Geometry: final body of the model. Coordinates: model frame, mm. Give positions to 0.01 mm unless a question says otherwise; leave off trailing zeros.
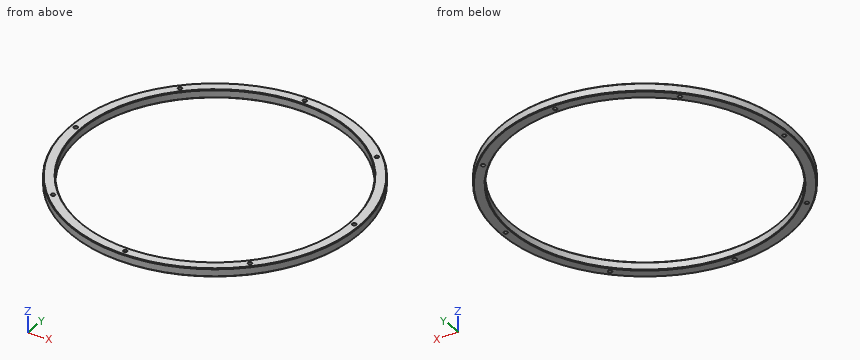
from build123d import *

# Parameters (mm, degrees)
SKETCH1_R             = 111.25
SKETCH1_R_2           = 103.25
EXTRUDE1_DEPTH        = 6.35
M3X0_5_TAPPED_HOLE1_D = 3
CIRPATTERN1_COUNT     = 8
CHAMFER1_SIZE         = 0.5


with BuildPart() as part:
    # Sketch1 → Extrude1 (new body)
    with BuildSketch(Plane.XY):
        Circle(SKETCH1_R)
        Circle(SKETCH1_R_2, mode=Mode.SUBTRACT)
    extrude(amount=EXTRUDE1_DEPTH)

    # M3x0.5 Tapped Hole1 (through all)
    with Locations(Plane.XY.offset(6.35)):
        with Locations((0, 107.125)):
            m3x0_5_tapped_hole1 = Hole(M3X0_5_TAPPED_HOLE1_D / 2)

    # CirPattern1: M3x0.5 Tapped Hole1 ×8 about axis
    cirpattern1_axis = Axis((0, 0, 0), (0, 0, 1))
    for i in range(1, CIRPATTERN1_COUNT):
        add(m3x0_5_tapped_hole1.rotate(cirpattern1_axis, i * 360 / CIRPATTERN1_COUNT), mode=Mode.SUBTRACT)

    # Chamfer1
    chamfer1_edges = [part.edges().sort_by_distance(p)[0] for p in [
        (-111.25, 0, 0),
        (-111.25, 0, 6.35),
        (-103.25, 0, 0),
        (-103.25, 0, 6.35),
    ]]
    chamfer(chamfer1_edges, length=CHAMFER1_SIZE)


solid = part.part
Q1. Section A-A on z = 4. Count the separate pieces of the cut face and the enclosed holes in it, plus the area to 3 significant figures.
Filled sheet:
separate pieces: 1
enclosed holes: 9
area: 5,330 mm2
Q2. Pin query (flat end, axial travel): P1, Ø1.8, axis at x = -107.125, y = 0, coming from the -Z side; P2, Ø1.5, axis at y = -9, z = 5, coming from the +X side; P3, Ø1.5, axis at x = -84.5, z = 4.5, coming from the -Y side. Return the tip coordinate at first contact, or that it passes through.
Filled sheet:
P1: passes through
P2: stops at x = 110.94
P3: stops at y = -73.23
Q3. Ray query, line 1 along Y through (x, z) = (0, 3.5) (3 decimals); line 2 along Y through (x, z) = (-77, 3.5); line 3 along X through (y, z) = (-0.5, 6). Return the intervals inside material, ascending.
Filled sheet:
line 1: y = -111.25 to -108.625, -105.625 to -103.25, 103.25 to 105.625, 108.625 to 111.25
line 2: y = -80.3 to -76.58, -74.92 to -68.79, 68.79 to 74.92, 76.58 to 80.3
line 3: x = -111.1 to -108.54, -105.71 to -103.4, 103.4 to 105.71, 108.54 to 111.1
